Work out the finished part from the listing and answer in its coordinate system (mm). Face numbers are marked on the shaded views. A direction names the side the tool comes from. Coordinates: 2 decimals unless noted, no trailing zeros. Loops run counter-clockwise (first coordinate to the right, second up) from the corner with the lowest first, then second, coordinate; pieces in that order, holes last.
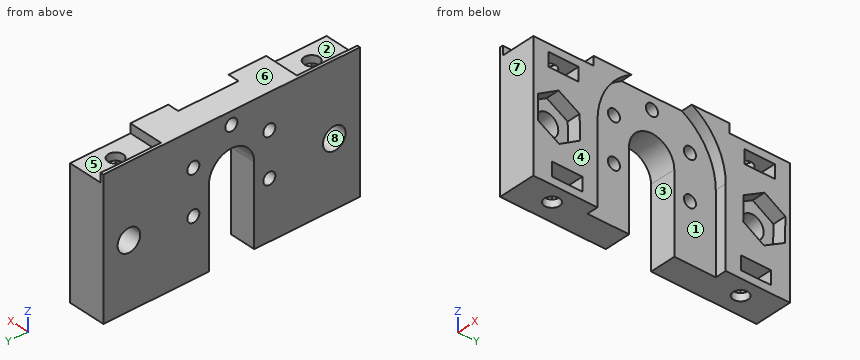
```python
from build123d import *

# Parameters (mm, degrees)
SKETCH_1_R          = 0.8
EXTRUDE_5_DEPTH     = 5
SKETCH_6_R          = 0.8
CUT_EXTRUDE_1_DEPTH = 1.5
SKETCH_7_R          = 1.5
CUT_EXTRUDE_2_DEPTH = 21.597329924
CUT_EXTRUDE_4_DEPTH = 1.8
SKETCH_9_R          = 1
CUT_EXTRUDE_5_DEPTH = 1
SKETCH_10_W         = 4
SKETCH_10_H         = 1.8
SKETCH_10_W_2       = 8
SKETCH_10_H_2       = 1.2
CUT_EXTRUDE_6_DEPTH = 4.6
SKETCH_12_R         = 1
CUT_EXTRUDE_7_DEPTH = 24.741103597


with BuildPart() as part:
    # ｽｹｯﾁ1 → ﾎﾞｽ - 押し出し5 (new body)
    # profile 1 of 3: a face of its own
    with BuildSketch(Plane.YZ):
        with BuildLine():
            Line((-3, -10.5), (-3, -7.95298686))
            ThreePointArc((-3, -7.95298686), (-8.482257997, -0.548907345), (-4, 7.5))
            Line((-4, 7.5), (-17, 7.5))
            Line((-17, 7.5), (-17, -10.5))
            Line((-17, -10.5), (-3, -10.5))
        make_face()
    # profile 2 of 3: a face of its own
    with BuildSketch(Plane.YZ):
        with BuildLine():
            ThreePointArc((-3, 0), (0, 3), (3, 0))
            Line((3, 0), (3, -7.95298686))
            ThreePointArc((3, -7.95298686), (6.991065727, -4.834769901), (8.5, 0))
            ThreePointArc((8.5, 0), (7.288689869, 4.373213921), (4, 7.5))
            Line((4, 7.5), (-4, 7.5))
            ThreePointArc((-4, 7.5), (-8.482257997, -0.548907345), (-3, -7.95298686))
            Line((-3, -7.95298686), (-3, 0))
        make_face()
        with Locations(Location((-5, -2.886751346, 0), (0, 0, 270))):
            Circle(SKETCH_1_R, mode=Mode.SUBTRACT)
        with Locations(Location((5.074182173, -2.886751346, 0), (0, 0, 270))):
            Circle(SKETCH_1_R, mode=Mode.SUBTRACT)
        with Locations(Location((-5, 2.929580443, 0), (0, 0, 270))):
            Circle(SKETCH_1_R, mode=Mode.SUBTRACT)
        with Locations(Location((5.074182173, 2.929580443, 0), (0, 0, 270))):
            Circle(SKETCH_1_R, mode=Mode.SUBTRACT)
        with Locations(Location((0.037091086, 5.837746338, 0), (0, 0, 270))):
            Circle(SKETCH_1_R, mode=Mode.SUBTRACT)
    # profile 3 of 3: a face of its own
    with BuildSketch(Plane.YZ):
        with BuildLine():
            ThreePointArc((8.5, 0), (6.991065727, -4.834769901), (3, -7.95298686))
            Line((3, -7.95298686), (3, -10.5))
            Line((3, -10.5), (17, -10.5))
            Line((17, -10.5), (17, 7.5))
            Line((17, 7.5), (4, 7.5))
            ThreePointArc((4, 7.5), (7.288689869, 4.373213921), (8.5, 0))
        make_face()
    extrude(amount=-EXTRUDE_5_DEPTH)

    # ｽｹｯﾁ6 → ｶｯﾄ - 押し出し1 (cut)
    # profile 1 of 5: a face of its own
    with BuildSketch(Plane.YZ):
        with BuildLine():
            ThreePointArc((-4, 7.5), (-7.288689869, 4.373213921), (-8.5, 0))
            Line((-8.5, 0), (-3, 0))
            ThreePointArc((-3, 0), (0, 3), (3, 0))
            Line((3, 0), (8.5, 0))
            ThreePointArc((8.5, 0), (7.288689869, 4.373213921), (4, 7.5))
            Line((4, 7.5), (-4, 7.5))
        make_face()
        with Locations(Location((-5, 2.929580443, 0), (0, 0, 270))):
            Circle(SKETCH_6_R, mode=Mode.SUBTRACT)
        with Locations(Location((5.074182173, 2.929580443, 0), (0, 0, 270))):
            Circle(SKETCH_6_R, mode=Mode.SUBTRACT)
        with Locations(Location((0.037091086, 5.837746338, 0), (0, 0, 270))):
            Circle(SKETCH_6_R, mode=Mode.SUBTRACT)
    # profile 2 of 5: a face of its own
    with BuildSketch(Plane.YZ):
        with BuildLine():
            Line((-3, 0), (-8.5, 0))
            ThreePointArc((-8.5, 0), (-6.991065727, -4.834769901), (-3, -7.95298686))
            Line((-3, -7.95298686), (-3, 0))
        make_face()
        with Locations(Location((-5, -2.886751346, 0), (0, 0, 270))):
            Circle(SKETCH_6_R, mode=Mode.SUBTRACT)
    # profile 3 of 5: a face of its own
    with BuildSketch(Plane.YZ):
        with BuildLine():
            Line((8.5, 0), (3, 0))
            Line((3, 0), (3, -7.95298686))
            ThreePointArc((3, -7.95298686), (6.991065727, -4.834769901), (8.5, 0))
        make_face()
        with Locations(Location((5.074182173, -2.886751346, 0), (0, 0, 270))):
            Circle(SKETCH_6_R, mode=Mode.SUBTRACT)
    # profile 4 of 5: a face of its own
    with BuildSketch(Plane.YZ):
        with BuildLine():
            ThreePointArc((8.5, 0), (6.991065727, -4.834769901), (3, -7.95298686))
            Line((3, -7.95298686), (3, -10.5))
            Line((3, -10.5), (8.5, -10.5))
            Line((8.5, -10.5), (8.5, 0))
        make_face()
    # profile 5 of 5: a face of its own
    with BuildSketch(Plane.YZ):
        with BuildLine():
            ThreePointArc((-3, -7.95298686), (-6.991065727, -4.834769901), (-8.5, 0))
            Line((-8.5, 0), (-8.5, -10.5))
            Line((-8.5, -10.5), (-3, -10.5))
            Line((-3, -10.5), (-3, -7.95298686))
        make_face()
    extrude(amount=-CUT_EXTRUDE_1_DEPTH, mode=Mode.SUBTRACT)

    # ｽｹｯﾁ7 → ｶｯﾄ - 押し出し2 (cut, through all)
    with BuildSketch(Plane(origin=(-5, 0, 0), x_dir=(0, -1, 0), z_dir=(-1, 0, 0))):
        with Locations(Location((-13.611024943, -1.95, 0), (0, 0, 90))):
            Circle(SKETCH_7_R)
        with Locations(Location((13.611024943, -1.95, 0), (0, 0, 270))):
            Circle(SKETCH_7_R)
    extrude(amount=-CUT_EXTRUDE_2_DEPTH, mode=Mode.SUBTRACT)

    # ｽｹｯﾁ8 → ｶｯﾄ - 押し出し4 (cut)
    with BuildSketch(Plane.YZ):
        Polygon((10.81922748, -3.513926764), (10.860725904, -0.314195857), (13.652523367, 1.249730908), (16.402822406, -0.386073236), (16.361323982, -3.585804143), (13.569526519, -5.149730908), align=None)
        Polygon((-10.860725904, -0.314195857), (-13.652523367, 1.249730908), (-16.402822406, -0.386073236), (-16.361323982, -3.585804143), (-13.569526519, -5.149730908), (-10.81922748, -3.513926764), align=None)
    extrude(amount=-CUT_EXTRUDE_4_DEPTH, mode=Mode.SUBTRACT)

    # ｽｹｯﾁ9 → ｶｯﾄ - 押し出し5 (cut)
    with BuildSketch(Plane(origin=(0, 0, -10.5), x_dir=(1, 0, 0), z_dir=(0, 0, -1))):
        with Locations(Location((-2.3, 12.508141571, 0), (0, 0, 180))):
            Circle(SKETCH_9_R)
        with Locations((-2.3, -12.508141571)):
            Circle(SKETCH_9_R)
    extrude(amount=-CUT_EXTRUDE_5_DEPTH, mode=Mode.SUBTRACT)

    # ｽｹｯﾁ10 → ｶｯﾄ - 押し出し6 (cut)
    with BuildSketch(Plane.YZ):
        with Locations((-12.5, -8.6)):
            Rectangle(SKETCH_10_W, SKETCH_10_H)
        with Locations((12.5, -8.6)):
            Rectangle(SKETCH_10_W, SKETCH_10_H)
        with Locations((-13, 4.4)):
            Rectangle(SKETCH_10_W, SKETCH_10_H)
        with Locations((13, 4.4)):
            Rectangle(SKETCH_10_W, SKETCH_10_H)
        with Locations((-13, 6.9)):
            Rectangle(SKETCH_10_W_2, SKETCH_10_H_2)
        with Locations((13, 6.9)):
            Rectangle(SKETCH_10_W_2, SKETCH_10_H_2)
    extrude(amount=-CUT_EXTRUDE_6_DEPTH, mode=Mode.SUBTRACT)

    # ｽｹｯﾁ12 → ｶｯﾄ - 押し出し7 (cut, through all)
    with BuildSketch(Plane(origin=(0, 0, 5.3), x_dir=(1, 0, 0), z_dir=(0, 0, -1))):
        with Locations(Location((-2.3, 13, 0), (0, 0, 180))):
            Circle(SKETCH_12_R)
        with Locations(Location((-2.3, -13, 0), (0, 0, 180))):
            Circle(SKETCH_12_R)
    extrude(amount=-CUT_EXTRUDE_7_DEPTH, mode=Mode.SUBTRACT)


solid = part.part
```
1. A cutting plane is placed at C-C, the plane z = -1.5. Give the vertices of the cut face in (x, y).
2. A cutting plane is placed at D-D, the plane z = 4.5. Give the vertices of the cut face in (x, y), then the cut area to 3 significant figures.
3. Each of these flat-tipped pins is pushed along its axis until it touches: P1, Ø1.3, axis at y = 0.04, z = 5.84, coming from the +X side; P2, Ø1.7, axis at y = -14.5, z = -3, coming from the +X side; P3, Ø6, axis at y = 1.5, z = 5.5, coming from the +X side; P4, Ø1.3, axis at y = -12, z = 7, coming from the +X side. Where does it stop, or does it pass through?
4. Determine the mould class of the marked faces 6, 7 and 8 for opening direction Y: released by +Y, released by -Y, zero draft, split by the parting line, or undercut.
5. A cutting plane is placed at B-B, the plane y = -5. Give the vertices of the cut face in (x, z).
6. Straight lines are drawn through the part: probe 1 along Y at (x, z) = (-1.2, -8); probe 2 along Y at (x, z) = (-2.3, 5.85); probe 3 along Y at (x, z) = (-3.35, 4). For each, find the intervals that lie inside material, in ascending order.
7. A cutting plane is placed at A-A, the plane y = 13. Count the separate pieces of the cut face and the enclosed holes in it, then the cut area to 3 significant figures.
8. For the marked faces 1, 2, 3, 4 and 5, determine the directions among +Z, -Z, +X, -X, +Y, -Y from which every point of the face is accessible in a straight line to the end or side of a thin tool.
Answers below:
1. outline: (-5, -17) - (0, -17) - (0, -16.39) - (-1.8, -16.39) - (-1.8, -15.04) - (-5, -15.04) - close; (-5, -12.18) - (-1.8, -12.18) - (-1.8, -10.85) - (0, -10.85) - (0, -8.5) - (-1.5, -8.5) - (-1.5, -3) - (-5, -3) - close; (-5, 3) - (-1.5, 3) - (-1.5, 8.5) - (0, 8.5) - (0, 10.85) - (-1.8, 10.85) - (-1.8, 12.18) - (-5, 12.18) - close; (-5, 15.04) - (-1.8, 15.04) - (-1.8, 16.39) - (0, 16.39) - (0, 17) - (-5, 17) - close
2. outline: (-5, -17) - (0, -17) - (0, -15) - (-4.6, -15) - (-4.6, -11) - (0, -11) - (0, -7.21) - (-1.5, -7.21) - (-1.5, 7.21) - (0, 7.21) - (0, 11) - (-4.6, 11) - (-4.6, 15) - (0, 15) - (0, 17) - (-5, 17) - close
2. area: 112 mm2
3. P1: passes through
3. P2: stops at x = -1.8
3. P3: stops at x = -1.5
3. P4: stops at x = -4.6
4. face 6: zero draft
4. face 7: released by -Y
4. face 8: undercut
5. outline: (-5, -10.5) - (-1.5, -10.5) - (-1.5, -3.69) - (-5, -3.69) - close; (-5, -2.09) - (-1.5, -2.09) - (-1.5, 2.13) - (-5, 2.13) - close; (-5, 3.73) - (-1.5, 3.73) - (-1.5, 6.87) - (0, 6.87) - (0, 7.5) - (-5, 7.5) - close
6. probe 1: y = -17 to -14.5, -10.5 to -8.5, 8.5 to 10.5, 14.5 to 17
6. probe 2: y = -17 to -14, -12 to -0.76, 0.84 to 12, 14 to 17
6. probe 3: y = -17 to -15, -11 to 11, 15 to 17
7. separate pieces: 4
7. enclosed holes: 0
7. area: 45.2 mm2
8. face 1: -Z, +X
8. face 2: +Z, +X, -Y
8. face 3: -Z, +X, -X
8. face 4: +Z, -Z, +X, +Y, -Y
8. face 5: +Z, +X, +Y
